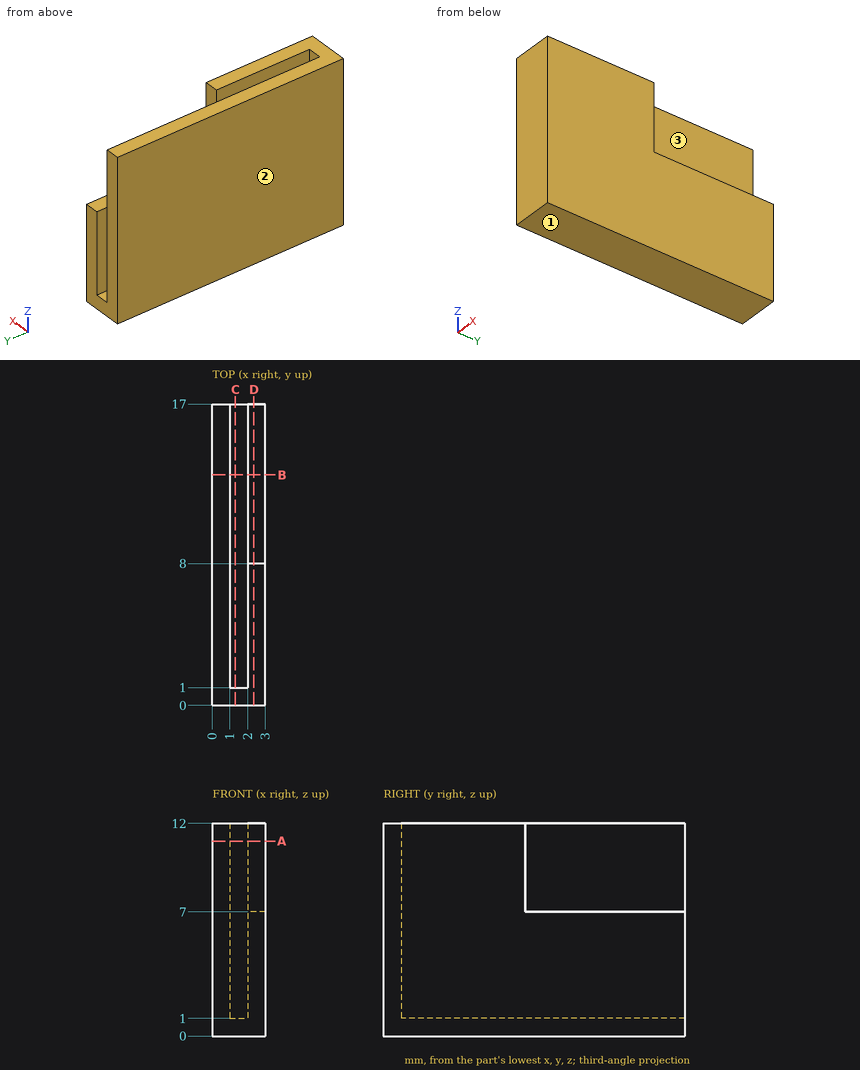
Here's the drawing with two shaded views (mm, measured from the low corner). I have some questions. Round coordinates to 2 decimals unless told otherwise and drop trailing zeros. Loops run counter-clockwise (first coordinate to the right, second up) from the corner with the lowest first, then second, coordinate; pieces in that order, holes last.
Item 1: Suppose I cut it at B-B, the plane y = 13. Write out the boundary of the cut face in (x, z).
Item 2: Will these pins go through, and if not, where does the flat tip stop? pin 1 Ø0.5 at (x, y) = (2.5, 11) entering from +Z; pin 2 Ø0.5 at (x, y) = (1.5, 12) entering from +Z.
Item 3: If we mould it in two halves opening along X, with no side actions, what happens to the marked faces 1, 2 and 3? For each: +X half, -X half, draft (parallel to the pull), parting line (faces both ways), or undercut.
Item 4: Suppose I cut it at A-A, the plane z = 11. Write out the boundary of the cut face in (x, y), then the cut area to 3 significant figures.
Item 5: Suppose I cut it at C-C, the plane x = 1.3. Write out the boundary of the cut face in (y, z).
Item 6: Suppose I cut it at D-D, the plane x = 2.35. Write out the boundary of the cut face in (y, z), then the cut area to 3 significant figures.
Item 7: Please list where these lines run through material, in increasing order: L1, parallel to X at y = 5.5, z = 7.5; L2, parallel to Y at x = 2.4, z = 8.25; L3, parallel to Y at x = 1.55, z = 5.25.
Reported:
1. outline: (0, 0) - (3, 0) - (3, 7) - (2, 7) - (2, 1) - (1, 1) - (1, 12) - (0, 12) - close
2. pin 1: stops at z = 7
2. pin 2: stops at z = 1
3. face 1: draft
3. face 2: -X half
3. face 3: undercut
4. outline: (0, 0) - (3, 0) - (3, 8) - (2, 8) - (2, 1) - (1, 1) - (1, 17) - (0, 17) - close
4. area: 26.0 mm2
5. outline: (0, 0) - (17, 0) - (17, 1) - (1, 1) - (1, 12) - (0, 12) - close
6. outline: (0, 0) - (17, 0) - (17, 7) - (8, 7) - (8, 12) - (0, 12) - close
6. area: 159 mm2
7. L1: x = 0 to 1, 2 to 3
7. L2: y = 0 to 8
7. L3: y = 0 to 1
